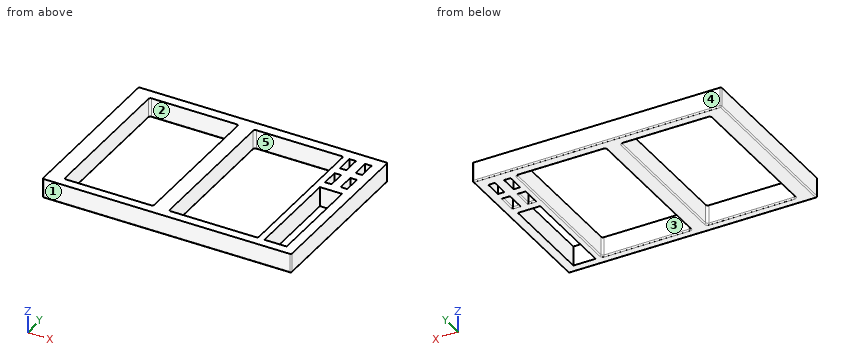
from build123d import *

# Parameters (mm, degrees)
ESQUISSE2_W        = 190
ESQUISSE2_H        = 130
ESQUISSE2_W_2      = 5
ESQUISSE2_H_2      = 13
ESQUISSE2_W_3      = 17
ESQUISSE2_H_3      = 74.885911828
BOSS_EXTRU_1_DEPTH = 15
CONG_1_R           = 1


with BuildPart() as part:
    # Esquisse2 → Boss.-Extru.1 (new body)
    with BuildSketch(Plane.XY):
        with Locations((229.947995903, -105.556817115)):
            Rectangle(ESQUISSE2_W, ESQUISSE2_H)
        with BuildLine():
            Line((294.126931092, -163.674733602), (229.09264334, -163.674733602))
            ThreePointArc((229.09264334, -163.674733602), (228.031983168, -163.235393774), (227.59264334, -162.174733602))
            Line((227.59264334, -162.174733602), (227.59264334, -49.858733602))
            ThreePointArc((227.59264334, -49.858733602), (228.031983168, -48.79807343), (229.09264334, -48.358733602))
            Line((229.09264334, -48.358733602), (294.126931092, -48.358733602))
            ThreePointArc((294.126931092, -48.358733602), (295.187591264, -48.79807343), (295.626931092, -49.858733602))
            Line((295.626931092, -49.858733602), (295.626931092, -162.174733602))
            ThreePointArc((295.626931092, -162.174733602), (295.187591264, -163.235393774), (294.126931092, -163.674733602))
        make_face(mode=Mode.SUBTRACT)
        with BuildLine():
            Line((214.126931092, -163.674733602), (149.09264334, -163.674733602))
            ThreePointArc((149.09264334, -163.674733602), (148.031983168, -163.235393774), (147.59264334, -162.174733602))
            Line((147.59264334, -162.174733602), (147.59264334, -49.858733602))
            ThreePointArc((147.59264334, -49.858733602), (148.031983168, -48.79807343), (149.09264334, -48.358733602))
            Line((149.09264334, -48.358733602), (214.126931092, -48.358733602))
            ThreePointArc((214.126931092, -48.358733602), (215.187591264, -48.79807343), (215.626931092, -49.858733602))
            Line((215.626931092, -49.858733602), (215.626931092, -162.174733602))
            ThreePointArc((215.626931092, -162.174733602), (215.187591264, -163.235393774), (214.126931092, -163.674733602))
        make_face(mode=Mode.SUBTRACT)
        with Locations((315.079916598, -55.443215784)):
            Rectangle(ESQUISSE2_W_2, ESQUISSE2_H_2, mode=Mode.SUBTRACT)
        with Locations((303.079916598, -55.443215784)):
            Rectangle(ESQUISSE2_W_2, ESQUISSE2_H_2, mode=Mode.SUBTRACT)
        with Locations((315.079916598, -75.443215784)):
            Rectangle(ESQUISSE2_W_2, ESQUISSE2_H_2, mode=Mode.SUBTRACT)
        with Locations((303.079916598, -75.443215784)):
            Rectangle(ESQUISSE2_W_2, ESQUISSE2_H_2, mode=Mode.SUBTRACT)
        with Locations((309.079916598, -126.231777688)):
            Rectangle(ESQUISSE2_W_3, ESQUISSE2_H_3, mode=Mode.SUBTRACT)
    extrude(amount=BOSS_EXTRU_1_DEPTH)

    # Congé1
    cong_1_edges = [part.edges().sort_by_distance(p)[0] for p in [
        (295.187591264, -163.235393774, 0),
        (295.626931092, -106.016733602, 0),
        (295.187591264, -48.79807343, 0),
        (261.609787216, -48.358733602, 0),
        (228.031983168, -48.79807343, 0),
        (227.59264334, -106.016733602, 0),
        (228.031983168, -163.235393774, 0),
        (261.609787216, -163.674733602, 0),
        (305.579916598, -75.443215784, 0),
        (303.079916598, -68.943215784, 0),
        (300.579916598, -75.443215784, 0),
        (303.079916598, -81.943215784, 0),
        (317.579916598, -75.443215784, 0),
        (315.079916598, -68.943215784, 0),
        (312.579916598, -75.443215784, 0),
        (315.079916598, -81.943215784, 0),
        (134.947995903, -105.556817115, 0),
        (229.947995903, -40.556817115, 0),
        (324.947995903, -105.556817115, 0),
        (229.947995903, -170.556817115, 0),
        (215.187591264, -163.235393774, 0),
        (215.626931092, -106.016733602, 0),
        (215.187591264, -48.79807343, 0),
        (181.609787216, -48.358733602, 0),
        (148.031983168, -48.79807343, 0),
        (147.59264334, -106.016733602, 0),
        (148.031983168, -163.235393774, 0),
        (181.609787216, -163.674733602, 0),
        (134.947995903, -170.556817115, 7.5),
        (134.947995903, -40.556817115, 7.5),
        (324.947995903, -40.556817115, 7.5),
        (324.947995903, -170.556817115, 7.5),
    ]]
    fillet(cong_1_edges, radius=CONG_1_R)


solid = part.part
Here's how the part is built. I have some questions about the finished solid (model axes, mm). Face numbers are marked on the shaded views. A direction names the side the tool comes from. Round coordinates to 2 decimals unless told otherwise and drop trailing zeros. Loops run counter-clockwise (first coordinate to the right, second up) from the corner with the lowest first, then second, coordinate; pieces in that order, holes last. Notation, with made-up numbers: (8, 31) - (36, 31) arc R17 ccw to (36, 63) - close; hole circle Ø6 at (-2, 75). An arc over 180 degrees is marked (long way). One line per question, with ' | ' between items. Start each with the question number.
Q1. I want a section at B-B (y = -75). State how many separate pieces and enclosed holes the cut face has, then the cut area to 3 significant figures.
Q2. We'd pull the mould along X, two halves only. Please class the marked faces 3, 4 and 5: +X half, -X half, draft (parallel to the pull), parting line (faces both ways), or undercut.
Q3. Please list where these lines run through material, in increasing order: line 1 (X direction, y = -55, z = 11.75); line 2 (X direction, y = -137.5, z = 7.25); line 3 (Y direction, x = 236.5, z = 3). Write a range as [from, to].
Q4. I want a section at A-A (x = 208). Write out the boundary of the cut face in (y, z).
Q5. I want a section at C-C (y = -91). Write out the boundary of the cut face in (x, z).
Q6. For the marked faces 1 and 2, which set-ups out of +Z, -Z, +X, -X, +Y, -Y let a thin tool reach every point of the face, with its end or its side?
Response values:
1) separate pieces: 5 | enclosed holes: 0 | area: 657 mm²
2) face 3: undercut | face 4: draft | face 5: undercut
3) line 1: x = [134.95, 147.59], [215.63, 227.59], [295.63, 300.58], [305.58, 312.58], [317.58, 324.95] | line 2: x = [134.95, 147.59], [215.63, 227.59], [295.63, 300.58], [317.58, 324.95] | line 3: y = [-170.56, -163.67], [-48.36, -40.56]
4) outline: (-170.56, 1) arc R1 ccw to (-169.56, 0) - (-164.67, 0) arc R1 ccw to (-163.67, 1) - (-163.67, 15) - (-170.56, 15) - close; (-48.36, 1) arc R1 ccw to (-47.36, 0) - (-41.56, 0) arc R1 ccw to (-40.56, 1) - (-40.56, 15) - (-48.36, 15) - close
5) outline: (134.95, 1) arc R1 ccw to (135.95, 0) - (146.59, 0) arc R1 ccw to (147.59, 1) - (147.59, 15) - (134.95, 15) - close; (215.63, 1) arc R1 ccw to (216.63, 0) - (226.59, 0) arc R1 ccw to (227.59, 1) - (227.59, 15) - (215.63, 15) - close; (295.63, 1) arc R1 ccw to (296.63, 0) - (300.58, 0) - (300.58, 15) - (295.63, 15) - close; (317.58, 0) - (323.95, 0) arc R1 ccw to (324.95, 1) - (324.95, 15) - (317.58, 15) - close
6) face 1: +Z, -Z, +X, -X, -Y | face 2: +Z, -Z
